The model under review builds one solid part; all positions refer to its coordinate system, in mm. Face numbers are marked on the shaded views. A direction names the side the tool comes from. Round coordinates to 2 decimals unless told otherwise and drop trailing zeros. Write each loop counter-clockwise with the first axis right and the second up, starting at its lowest first coordinate (ties: lowest second). Pieces come first, ordered by that corner, then holes. Notation, with made-up numbers: (70.25, -25) - (122.25, -25) arc R21 ccw to (122.25, -14) - close; hole circle Ø3 at (-22.5, 37.25). An arc over 180 degrees is marked (long way). Return JSON: item names as keys, results as strings.
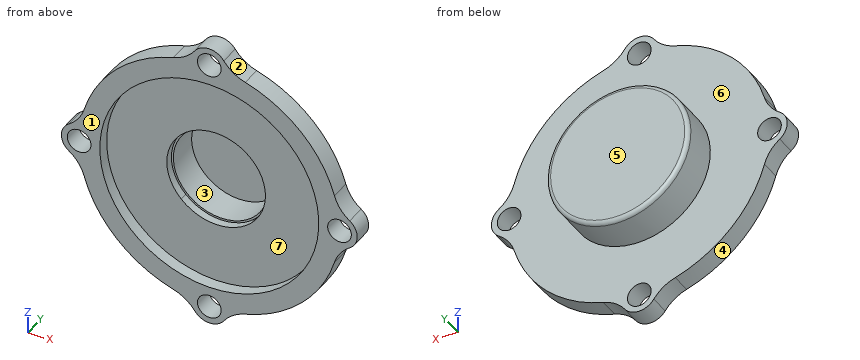
from build123d import *

# Parameters (mm, degrees)
BOSS_EXTRUDE1_OUTLINE_W = 75
BOSS_EXTRUDE1_OUTLINE_H = 75
BOSS_EXTRUDE1_OUTLINE_R = 3
BOSS_EXTRUDE1_DEPTH     = 5
SKETCH2_R               = 27.75
CUT_EXTRUDE1_DEPTH      = 3
SKETCH3_OUTSIDE_W       = 98.236
SKETCH3_OUTSIDE_H       = 98.236
CUT_EXTRUDE5_DEPTH      = 5
SKETCH4_R               = 18
BOSS_EXTRUDE2_DEPTH     = 9.5
SKETCH5_R               = 12
CUT_EXTRUDE6_DEPTH      = 8
FILLET1_R               = 1


# Read off the part's stored shape, not the designer's step: Boss-Extrude1
with BuildPart() as part:
    # Boss-Extrude1 outline → Boss-Extrude1 (new body)
    with BuildSketch(Plane(origin=(0, 0, 0), x_dir=(1, 0, 0), z_dir=(0, 1, 0))):
        Rectangle(BOSS_EXTRUDE1_OUTLINE_W, BOSS_EXTRUDE1_OUTLINE_H)
        with Locations((0.001, -33.001)):
            Circle(BOSS_EXTRUDE1_OUTLINE_R, mode=Mode.SUBTRACT)
        with Locations((-33, 0)):
            Circle(BOSS_EXTRUDE1_OUTLINE_R, mode=Mode.SUBTRACT)
        with BuildLine():
            ThreePointArc((8.840334751, 8.839334751), (12.502, 0), (8.840334751, -8.839334751))
            ThreePointArc((8.840334751, -8.839334751), (0.001, -12.501), (-8.838334751, -8.839334751))
            ThreePointArc((-8.838334751, -8.839334751), (-12.5, 0), (-8.838334751, 8.839334751))
            ThreePointArc((-8.838334751, 8.839334751), (0.001, 12.501), (8.840334751, 8.839334751))
        make_face(mode=Mode.SUBTRACT)
        with Locations((33.002, 0)):
            Circle(BOSS_EXTRUDE1_OUTLINE_R, mode=Mode.SUBTRACT)
        with Locations((0.001, 33.001)):
            Circle(BOSS_EXTRUDE1_OUTLINE_R, mode=Mode.SUBTRACT)
    extrude(amount=BOSS_EXTRUDE1_DEPTH)

    # Sketch2 → Cut-Extrude1 (cut)
    with BuildSketch(Plane.XZ):
        with Locations(Location((0, 0, 0), (0, 0, 270))):
            Circle(SKETCH2_R)
    extrude(amount=-CUT_EXTRUDE1_DEPTH, mode=Mode.SUBTRACT)

    # Sketch3 outside → Cut-Extrude5 (cut)
    with BuildSketch(Plane.XZ):
        Rectangle(SKETCH3_OUTSIDE_W, SKETCH3_OUTSIDE_H)
        with BuildLine():
            ThreePointArc((-31.718023256, -9.10862233), (-23.334523779, -23.334523779), (-9.10862233, -31.718023256))
            ThreePointArc((-9.10862233, -31.718023256), (-6.064515675, -33.186440594), (-3.683424077, -35.585031348))
            ThreePointArc((-3.683424077, -35.585031348), (0, -37.5), (3.683424077, -35.585031348))
            ThreePointArc((3.683424077, -35.585031348), (6.064515675, -33.186440594), (9.10862233, -31.718023256))
            ThreePointArc((9.10862233, -31.718023256), (23.334523779, -23.334523779), (31.718023256, -9.10862233))
            ThreePointArc((31.718023256, -9.10862233), (33.186440594, -6.064515675), (35.585031348, -3.683424077))
            ThreePointArc((35.585031348, -3.683424077), (37.5, 0), (35.585031348, 3.683424077))
            ThreePointArc((35.585031348, 3.683424077), (33.186440594, 6.064515675), (31.718023256, 9.10862233))
            ThreePointArc((31.718023256, 9.10862233), (23.334523779, 23.334523779), (9.10862233, 31.718023256))
            ThreePointArc((9.10862233, 31.718023256), (6.064515675, 33.186440594), (3.683424077, 35.585031348))
            ThreePointArc((3.683424077, 35.585031348), (0, 37.5), (-3.683424077, 35.585031348))
            ThreePointArc((-3.683424077, 35.585031348), (-6.064515675, 33.186440594), (-9.10862233, 31.718023256))
            ThreePointArc((-9.10862233, 31.718023256), (-23.334523779, 23.334523779), (-31.718023256, 9.10862233))
            ThreePointArc((-31.718023256, 9.10862233), (-33.186440594, 6.064515675), (-35.585031348, 3.683424077))
            ThreePointArc((-35.585031348, 3.683424077), (-37.5, 0), (-35.585031348, -3.683424077))
            ThreePointArc((-35.585031348, -3.683424077), (-33.186440594, -6.064515675), (-31.718023256, -9.10862233))
        make_face(mode=Mode.SUBTRACT)
    extrude(amount=-CUT_EXTRUDE5_DEPTH, mode=Mode.SUBTRACT)

    # Sketch4 → Boss-Extrude2 (add)
    with BuildSketch(Plane(origin=(0, 5, 0), x_dir=(1, 0, 0), z_dir=(0, 1, 0))):
        with Locations(Location((0, 0.647401089, 0), (0, 0, 270))):
            Circle(SKETCH4_R)
    extrude(amount=BOSS_EXTRUDE2_DEPTH)

    # Sketch5 → Cut-Extrude6 (cut)
    with BuildSketch(Plane.XZ.offset(-5)):
        with Locations(Location((0, 0, 0), (0, 0, 270))):
            Circle(SKETCH5_R)
    extrude(amount=-CUT_EXTRUDE6_DEPTH, mode=Mode.SUBTRACT)

    # Fillet1
    fillet1_edges = [part.edges().sort_by_distance(p)[0] for p in [
        (0, 14.5, -18.647401089),
    ]]
    fillet(fillet1_edges, radius=FILLET1_R)


solid = part.part
(1) For the marked faces 5, 6 and 7, list the 3-axis set-ups (+Z, -Z, +X, -X, +Y, -Y) from which the entire face can be reached by the end or side of a thin tool; tool diameter is ignored.
Filled in:
{"face 5": "+Z, -Z, +X, -X, +Y", "face 6": "+Y", "face 7": "-Y"}
(2) Add section C-C (x = -33). Write out the cut boundary in (y, z).
Filled in:
{"outline": "(0, -6.34) - (5, -6.34) - (5, -3) - (0, -3) - close; (0, 3) - (5, 3) - (5, 6.34) - (0, 6.34) - close"}
(3) Add section B-B (y = 6). Write out the cut boundary in (x, z), plus the area to 3 significant figures.
Filled in:
{"outline": "circle Ø36 at (0, -0.65); hole circle Ø24 at (0, 0)", "area": "565 mm2"}
(4) Clearance check with flat-ended pins moving along their axes: pin 1 Ø1.5 at (y, z) = (4.5, 23.5) entering from +X; pin 2 Ø16.5 at (x, z) = (-11, 3.5) entering from -Y; pin 3 Ø2 at (x, z) = (-24, 5) entering from +Y; pin 4 Ø3 at (y, z) = (7.5, 26.5) entering from +X. State where each tip first meets the part, or that it passes through.
Filled in:
{"pin 1": "stops at x = 23.9", "pin 2": "stops at y = 3", "pin 3": "stops at y = 5", "pin 4": "passes through"}
(5) Wall thickness on line 1 (X direction, y = 2.7, z = 0); line 2 (X direction, y = 7.5, z = 0); line 3 (X direction, y = 3.8, z = 0): over which ranges is each line inside the solid? List them lowest first.
Filled in:
{"line 1": "x = -37.5 to -36, -30 to -27.75, 27.75 to 30, 36 to 37.5", "line 2": "x = -17.99 to -12, 12 to 17.99", "line 3": "x = -37.5 to -36, -30 to -12.5, 12.5 to 30, 36 to 37.5"}
(6) Add section A-A (x = 0). Give the number of separate pieces and of enclosed holes in the cut face, plus the area to 3 significant figures.
Filled in:
{"separate pieces": "3", "enclosed holes": "0", "area": "248 mm2"}
(7) Mouldability with a two-part tool opening along Z and no side actions: class the marked faces 1, 2, 3 and 4 as released by +Z, released by -Z, zero draft, split by the parting line, or undercut.
Filled in:
{"face 1": "zero draft", "face 2": "released by +Z", "face 3": "undercut", "face 4": "released by -Z"}
